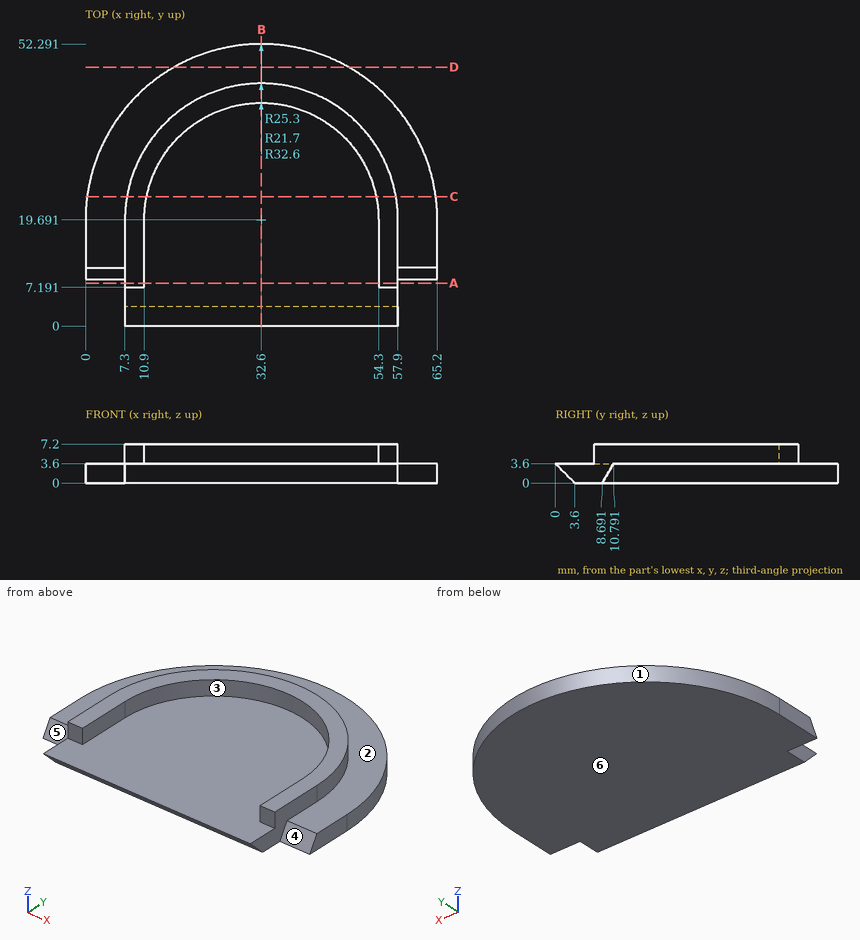
Job drawing, mm, ordinate dimensions from the low corner. One solid piece. A direction names the side the tool comes from. Round coordinates to 2 decimals unless told otherwise and drop trailing zeros. Write each loop counter-clockwise with the first axis right and the second up, starting at its lowest first coordinate (ties: lowest second). Pieces come first, ordered by that corner, then holes. Notation, with made-up numbers: M -22.5,23 L -9.5,23 A18 ccw -9.5,28 Z; hole C 89.25,83 d4. An arc over 180 degrees is marked long. Return JSON: item names as keys, results as strings. Group by question number.
(1) Saw through at D-D on y = 48. Write the cut outline in (x, z), then the cut area to 3 significant figures.
(2) Two-plate mould, pull along X, no slides. Class the marked faces 1, 2 and 3: +X half, -X half, draft (parallel to the pull), parting line (faces both ways), or undercut.
(3) Drill centre lines: probe 1 along X at (y, z) = (15.5, 5.5); probe 2 along X at (y, z) = (2, 1.75); probe 3 along Z at (x, y) = (26, 8.5). Where is each one in solid material? Low to high.
(4) Pin check, flat tips, straight feed: pin 1 Ø1.1 at (y, z) = (12, 5) entering from +X; pin 2 Ø1.5 at (y, z) = (37.5, 5) entering from +X; pin 3 Ø20.5 at (x, y) = (38.5, 26) entering from +Z. Stop position of each tip, or through.
(5) Which spindle directions (+Z, -Z, +X, -X, +Y, -Y) get a long thin tool onto all of the face, cutting with end or side? Do the marked faces 4, 5 and 6. Say none if no direction does.
(6) Saw through at B-B on x = 32.6. Write the cut outline in (y, z), then the cut area to 3 significant figures.
(7) Saw through at C-C on y = 24. Write the cut outline in (x, z), then the cut area to 3 significant figures.
(8) Saw through at A-A on y = 8. Write the cut outline in (x, z), then the cut area to 3 significant figures.
Returned:
{
 "1": {"outline": "M 16.43,0 L 48.77,0 L 48.77,3.6 L 16.43,3.6 Z", "area": "116 mm²"},
 "2": {"face 1": "parting line", "face 2": "draft", "face 3": "undercut"},
 "3": {"probe 1": "7.3 to 10.9, 54.3 to 57.9", "probe 2": "7.3 to 57.9", "probe 3": "0 to 3.6"},
 "4": {"pin 1": "x = 57.9", "pin 2": "x = 51.28", "pin 3": "z = 3.6"},
 "5": {"face 4": "+Z, +X, -Y", "face 5": "+Z, -X, -Y", "face 6": "-Z, +X, -X, +Y, -Y"},
 "6": {"outline": "M 0,3.6 L 3.6,0 L 52.29,0 L 52.29,3.6 L 44.99,3.6 L 44.99,7.2 L 41.39,7.2 L 41.39,3.6 Z", "area": "195 mm²"},
 "7": {"outline": "M 0.29,0 L 64.91,0 L 64.91,3.6 L 57.53,3.6 L 57.53,7.2 L 53.87,7.2 L 53.87,3.6 L 11.33,3.6 L 11.33,7.2 L 7.67,7.2 L 7.67,3.6 L 0.29,3.6 Z", "area": "259 mm²"},
 "8": {"outline": "M 7.3,0 L 57.9,0 L 57.9,7.2 L 54.3,7.2 L 54.3,3.6 L 10.9,3.6 L 10.9,7.2 L 7.3,7.2 Z", "area": "208 mm²"}
}
